Can you work these out from the model? Positions are in its coordinate system, mm. Face numbers are marked on the shaded views. Coordinates: 2 decimals unless noted, no trailing zeros. Loops run counter-clockwise (first coordinate to the right, second up) from the corner with the lowest first, then second, coordinate; pieces in that order, holes last. Notation, with made-up numbers: M 80,10 L 115,10 A12 cw 115,16 Z; hole C 49,-38 d7. An arc over 180 degrees is marked long. Answer as a JSON object with one key per item and string values. Group by question number.
Item 1: We'd pull the mould along Y, two halves only. Please class the marked faces 1, 2 and 3: +Y half, -Y half, draft (parallel to the pull), parting line (faces both ways), or undercut.
Item 2: Suppose I cut it at A-A (z = 4.5). Write out the boundary of the cut face in (x, y), then the cut area to 3 significant figures.
Item 3: I'm going to push flat-ended pins straight in: pin 1 Ø12 at (x, y) = (57.5, -6.5) entering from -Z; pin 2 Ø2 at (x, z) = (116.5, 12) entering from -Y; pin 3 Ø1 at (x, y) = (45, -98.5) entering from -Z. Where does each tip first touch, or does it pass through?
Item 4: If I drill on line 1 (Z direction, x = 127, y = 16); line 2 (Z direction, x = 121.5, y = -89.5), over which ranges is the centre line in solid material (lowest first)?
Item 5: Suppose I cut it at B-B (x = 65). Write out the boundary of the cut face in (y, z).
Item 6: Suppose I cut it at C-C (y = 18). Write out the boundary of the cut face in (x, z), then the cut area to 3 significant figures.
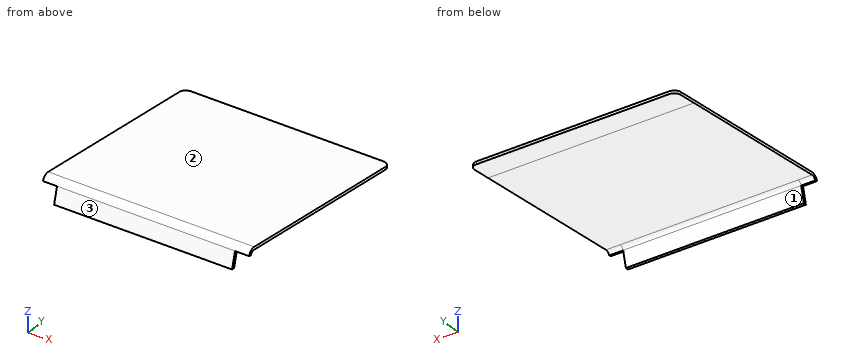
```python
from build123d import *

# Parameters (mm, degrees)
F3_DEPTH  = 131
F4_T      = -2
F5_DEPTH  = 2
F6_DEPTH  = 2
F7_DEPTH  = 2
F9_DEPTH  = 127
F13_DEPTH = 10
F15_DEPTH = 10
F16_R     = 5


with BuildPart() as f3:
    # F2 (on Right) → F3 (new body)
    with BuildSketch(Plane.YZ):
        with BuildLine():
            ThreePointArc((-91.0913455441, 16.9367446821), (-94.4482121177, 16.0862273851), (-96.4473620115, 13.2586254741))
            Line((-96.4473620115, 13.2586254741), (-100, 0))
            Line((-100, 0), (50, 0))
            Line((50, 0), (50, 2))
            Line((50, 2), (-91.0913455441, 16.9367446821))
        make_face()
    extrude(amount=F3_DEPTH)

    # F4 (hollow: no face is removed)
    offset(amount=F4_T, mode=Mode.SUBTRACT)

    # F5 (cut): a face of the model
    f5_faces = [f3.faces().sort_by_distance(p)[0] for p in [
        (65.5, -25, 0),
    ]]
    extrude(f5_faces, amount=-F5_DEPTH, mode=Mode.SUBTRACT)

    # F6 (cut): a face of the model
    f6_faces = [f3.faces().sort_by_distance(p)[0] for p in [
        (131, -48.1192247529, 7.0991070321),
    ]]
    extrude(f6_faces, amount=-F6_DEPTH, mode=Mode.SUBTRACT)

    # F7 (cut): a face of the model
    f7_faces = [f3.faces().sort_by_distance(p)[0] for p in [
        (0, -48.1192247529, 7.0991070321),
    ]]
    extrude(f7_faces, amount=-F7_DEPTH, mode=Mode.SUBTRACT)


with BuildPart() as f9:
    # F8 (on face) → F9 (new body)
    with BuildSketch(Plane.YZ.offset(129)):
        Polygon((50, 2), (31.0025824745, 2), (50, 0), align=None)
    extrude(amount=-F9_DEPTH)

    # F10: union F3
    add(f3.part)

    # F12 (on face) → F13 (join)
    with BuildSketch(Plane.YZ.offset(129)):
        Polygon((50, 2), (-91.0913455441, 16.9367446821), (-91.3019004785, 14.9478589087), (31.0025824745, 2), (50, 0), align=None)
        with BuildLine():
            ThreePointArc((-91.0913455441, 16.9367446821), (-94.4482121177, 16.0862273851), (-96.4473620115, 13.2586254741))
            Line((-96.4473620115, 13.2586254741), (-94.5155103589, 12.7409873839))
            ThreePointArc((-94.5155103589, 12.7409873839), (-93.3160204226, 14.4375485305), (-91.3019004785, 14.9478589087))
            Line((-91.3019004785, 14.9478589087), (-91.0913455441, 16.9367446821))
        make_face()
    extrude(amount=F13_DEPTH)

    # F14 (on face) → F15 (join)
    with BuildSketch(Plane(origin=(2, 0, 0), x_dir=(0, -1, 0), z_dir=(-1, 0, 0))):
        with BuildLine():
            ThreePointArc((91.3019004785, 14.9478589087), (93.3160204226, 14.4375485305), (94.5155103589, 12.7409873839))
            Line((94.5155103589, 12.7409873839), (96.4473620115, 13.2586254741))
            ThreePointArc((96.4473620115, 13.2586254741), (94.4482121177, 16.0862273851), (91.0913455441, 16.9367446821))
            Line((91.0913455441, 16.9367446821), (-50, 2))
            Line((-50, 2), (-50, 0))
            Line((-50, 0), (-31.0025824745, 2))
            Line((-31.0025824745, 2), (91.3019004785, 14.9478589087))
        make_face()
    extrude(amount=F15_DEPTH)

    # F16
    f16_edges = [f9.edges().sort_by_distance(p)[0] for p in [
        (139, 50, 1),
        (-8, 50, 1),
    ]]
    fillet(f16_edges, radius=F16_R)


solid = f9.part
```
From the geometry:
{
 "1": {"face 1": "undercut", "face 2": "+Y half", "face 3": "-Y half"},
 "2": {"outline": "M -8,7.39 L 139,7.39 L 139,26.39 L -8,26.39 Z; M 2,-98.79 L 129,-98.79 L 129,-96.72 L 2,-96.72 Z", "area": "3,060 mm2"},
 "3": {"pin 1": "z = 5.34", "pin 2": "y = -97.05", "pin 3": "z = 2"},
 "4": {"line 1": "3.59 to 5.6", "line 2": "14.76 to 16.77"},
 "5": {"outline": "M -99.46,2 L -97.39,2 L -94.52,12.74 A3 cw -91.3,14.95 L 31,2 L 50,0 L 50,2 L -91.09,16.94 A5 ccw -96.45,13.26 Z"},
 "6": {"outline": "M -8,3.38 L 139,3.38 L 139,5.39 L -8,5.39 Z", "area": "296 mm2"}
}
